from build123d import *

# Parameters (mm, degrees)
SZKIC1_R = 8


with BuildPart() as part:
    # Szkic2 → Obrót1 (revolve)
    with BuildSketch(Plane.XY, mode=Mode.PRIVATE) as obr_t1_sk:
        with BuildLine():
            Line((0, 14), (16.942496363, 14))
            ThreePointArc((16.942496363, 14), (18.293676778, 13.474554674), (18.934885759, 12.174311485))
            Line((18.934885759, 12.174311485), (20, 0))
            Line((20, 0), (0, 0))
            Line((0, 0), (0, 14))
        make_face()
    revolve(obr_t1_sk.sketch.rotate(Axis((0, 0, 0), (0, 1, 0)), 270), axis=Axis((0, 0, 0), (0, 1, 0)))

    # Szkic1 → Obrót2 (revolve)
    with BuildSketch(Plane(origin=(0, 0, 0), x_dir=(0, 0, -1), z_dir=(1, 0, 0)), mode=Mode.PRIVATE) as obr_t2_sk:
        with Locations((0, 62)):
            Circle(SZKIC1_R)
    revolve(obr_t2_sk.sketch.rotate(Axis((0, 35, -8), (0, 0, 1)), 26.239647144), axis=Axis((0, 35, -8), (0, 0, 1)))

    # Szkic3 → Obrót3 (revolve)
    with BuildSketch(Plane.XY, mode=Mode.PRIVATE) as obr_t3_sk:
        Polygon((0, 0), (10, 0), (10, -28.4665), (8.4665, -30), (0, -30), align=None)
    revolve(obr_t3_sk.sketch.rotate(Axis((0, -30, 0), (0, 1, 0)), 270), axis=Axis((0, -30, 0), (0, 1, 0)))

    # Szkic4 → Wycięcie-obrót1 (revolve, cut)
    with BuildSketch(Plane.XY, mode=Mode.PRIVATE) as wyci_cie_obr_t1_sk:
        Polygon((9, 0), (9, -3), (10, -4), (10, 0), align=None)
    revolve(wyci_cie_obr_t1_sk.sketch.rotate(Axis((0, -30, 0), (0, 1, 0)), 270), axis=Axis((0, -30, 0), (0, 1, 0)), mode=Mode.SUBTRACT)


solid = part.part
Design review of the part built by this model. Coordinates are the model's own, in mm. A direction names the side the tool comes from. Give positions to 0.01 mm unless a question says otherwise; leave off trailing zeros. Order: outer loops, then holes, each group sorted by start corner. A loop starts at its lowest first (then second) coordinate and runs counter-clockwise, first axis right, second up. Notation, with made-up numbers: (78.5, 43.25) - (102.5, 43.25) arc R27 cw to (102.5, 75.25) - close; hole circle Ø2 at (11.25, -33.5). An arc over 180 degrees is marked (long way). Write item = value, one per line. Start each with the question number.
Q1. Mouldability with a two-part tool opening along Y and no side actions: class faces 1 (the face through (-9.76, -16.4, -2.17)), 2 (the face through (0, -30, 0)), 3 (the face through (2.703, -1.521, 8.584)) as released by +Y, released by -Y, zero draft, split by the parting line, or undercut.
Q2. Tool access review of faces 4 (the face through (5.814, 7.355, 18.463)), 5 (the face through (0, 14, 11)), 6 (the face through (0, 14, -11)): name each direction out of +Z, -Z, +X, -X, +Y, -Y from which nothing blocks a thin tool from reaching the whole face with its end or side.
Q3. We need section B-B on z = 0. State the section outline as (x, y) points.
Q4. Clearance check with flat-ended pins moving along their axes: pin 1 Ø2 at (x, z) = (2.5, 10.5) entering from -Y; pin 2 Ø10 at (x, y) = (20.5, 43) entering from -Z; pin 3 Ø3 at (x, y) = (8, 59.5) entering from +Z. State where each tip first meets the part, or that it passes through.
Q5. We need section A-A on x = 0. State the section outline as (y, z) points.
Q6. We need section C-C on y = -22.5. State the section outline as (x, z) points.
Q7. To check wall thickness, follow L1, parallel to Y at x = 16, z = 0; L2, parallel to X at y = -8, z = -6; L3, parallel to Y at x = -15, z = 2.5. State the ranges of each line that lie inside material, in increasing order. Write a range as from..to.
Working result:
q1.face_1 = zero draft
q1.face_2 = released by -Y
q1.face_3 = undercut
q2.face_4 = none
q2.face_5 = +Z
q2.face_6 = -Z
q3.outline = (-20, 0) - (-9, 0) - (-9, -3) - (-10, -4) - (-10, -28.47) - (-8.47, -30) - (8.47, -30) - (10, -28.47) - (10, -4) - (9, -3) - (9, 0) - (20, 0) - (19.48, 5.92) arc R35 ccw (long way) to (-19.48, 5.92) - close; hole circle Ø38 at (0, 35)
q4.pin_1 = -28.67
q4.pin_2 = -8
q4.pin_3 = 8
q5.outline = (-30, -8.47) - (-28.47, -10) - (-4, -10) - (-3, -9) - (0, -9) - (0, -20) - (12.17, -18.93) arc R2 ccw to (14, -16.94) - (14, -5.29) arc R8 ccw to (14, 5.29) - (14, 16.94) arc R2 ccw to (12.17, 18.93) - (0, 20) - (0, 9) - (-3, 9) - (-4, 10) - (-28.47, 10) - (-30, 8.47) - close; circle Ø16 at (62, 0)
q6.outline = circle Ø20 at (0, 0)
q7.L1 = 0..24.75, 45.25..66.13
q7.L2 = -8..8
q7.L3 = 0..22.7, 47.3..66.18
